```python
from build123d import *

# Parameters (mm, degrees)
SKETCH1_W           = 40
SKETCH1_H           = 650
BOSS_EXTRUDE1_DEPTH = 3.175
SKETCH2_R           = 14.279
CUT_EXTRUDE1_DEPTH  = 4.175


with BuildPart() as part:
    # Sketch1 → Boss-Extrude1 (new body)
    with BuildSketch(Plane.XY):
        with Locations((20, -325)):
            Rectangle(SKETCH1_W, SKETCH1_H)
    extrude(amount=BOSS_EXTRUDE1_DEPTH)

    # Sketch2 → Cut-Extrude1 (cut, through all)
    with BuildSketch(Plane.XY.offset(3.175)):
        with Locations((20, -18.141364063)):
            Circle(SKETCH2_R)
        with Locations((20, -630)):
            Circle(SKETCH2_R)
        with Locations((20, -300)):
            Circle(SKETCH2_R)
    extrude(amount=-CUT_EXTRUDE1_DEPTH, mode=Mode.SUBTRACT)


solid = part.part
```
Geometry: final body of the model. Coordinates: model frame, mm. Give positions to 0.01 mm unless a question says otherwise; leave off trailing zeros. Order: outer loops, then holes, each group sorted by start corner. A loop starts at its lowest first (then second) coordinate and runs counter-clockwise, first axis right, second up. Notation, with made-up numbers: M 81.25,-3 L 127.25,-3 A11 ccw 127.25,6 Z; hole C -10,30.25 d7. An arc over 180 degrees is marked long. Answer as CSV lines item,"result". Start each with the question number.
1) Cut plane B-B (x = 20). Output: boundary loops of the cut face in (y, z) (3 decimals), then the cut area to 3 significant figures.
2) Line query: line 1 (Y direction, x = 20, z = 1.35); line 2 (Y direction, x = 21, z = 0.75); line 3 (X direction, y = -630, z = 1). Output: solid intervals per line, ascending. Write a range as from..to.
3) Cut plane C-C (z = 2.3). Output: boundary loops of the cut face in (x, y), then the cut area to 3 significant figures.
4) Cut plane A-A (y = -630). Output: boundary loops of the cut face in (x, z) (3 decimals), then the cut area to 3 significant figures.
5) Mould query, pull axis Y, two halves, no side actions, for faces 1 (the cylindrical face through (16.9, -313.94, 1.61)), 2 (the flat face through (20, -320, 0)). Classes: +Y half, -Y half, draft (parallel to the pull), parting line (faces both ways), or undercut.
Findings below:
1,outline,"M -650,0 L -644.279,0 L -644.279,3.175 L -650,3.175 Z; M -615.721,0 L -314.279,0 L -314.279,3.175 L -615.721,3.175 Z; M -285.721,0 L -32.42,0 L -32.42,3.175 L -285.721,3.175 Z; M -3.862,0 L 0,0 L 0,3.175 L -3.862,3.175 Z"
1,area,"1,790 mm²"
2,line 1,"y = -650..-644.28, -615.72..-314.28, -285.72..-32.42, -3.86..0"
2,line 2,"y = -650..-644.24, -615.76..-314.24, -285.76..-32.39, -3.9..0"
2,line 3,"x = 0..5.72, 34.28..40"
3,outline,"M 0,-650 L 40,-650 L 40,0 L 0,0 Z; hole C 20,-630 d28.56; hole C 20,-300 d28.56; hole C 20,-18.14 d28.56"
3,area,"24,100 mm²"
4,outline,"M 0,0 L 5.721,0 L 5.721,3.175 L 0,3.175 Z; M 34.279,0 L 40,0 L 40,3.175 L 34.279,3.175 Z"
4,area,"36.3 mm²"
5,face 1,"undercut"
5,face 2,"draft"
